from build123d import *

# Parameters (mm, degrees)
SKETCH1_W       = 34.29
SKETCH1_H       = 34.29
EXTRUDE1_DEPTH  = 1.27
SKETCH2_R       = 1.27
EXTRUDE2_DEPTH  = 2.27
SKETCH3_R       = 0.9525
EXTRUDE3_DEPTH  = 2.27
SKETCH4_R       = 0.5715
EXTRUDE4_DEPTH  = 2.27
LPATTERN1_COUNT = 3
LPATTERN1_PITCH = 2.54
SKETCH5_R       = 0.508
EXTRUDE5_DEPTH  = 2.27
LPATTERN2_COUNT = 8
LPATTERN2_PITCH = 2.54
SKETCH7_W       = 7.030885781
SKETCH7_H       = 5.062237762
SKETCH7_W_2     = 7.874
SKETCH7_H_2     = 7.62
SKETCH7_W_3     = 3.281080031
SKETCH7_H_3     = 6.374669774
SKETCH7_W_4     = 3.421697746
SKETCH7_H_4     = 4.921620047
SKETCH7_W_5     = 2.577991453
SKETCH7_H_5     = 1.453049728
SKETCH7_W_6     = 3.140462315
SKETCH7_H_6     = 1.406177157
SKETCH7_W_7     = 3.327952603
SKETCH7_H_7     = 1.078069153
EXTRUDE7_DEPTH  = 1.27
SKETCH8_R       = 3.175
EXTRUDE8_DEPTH  = 5.08
SKETCH9_W       = 7.112
SKETCH9_H       = 8.89
EXTRUDE9_DEPTH  = 2.54


with BuildPart() as part:
    # Sketch1 → Extrude1 (new body)
    with BuildSketch(Plane.XY):
        Rectangle(SKETCH1_W, SKETCH1_H)
    extrude(amount=EXTRUDE1_DEPTH)

    # Sketch2 → Extrude2 (cut, through all)
    with BuildSketch(Plane.XY.offset(1.27)):
        with Locations((-14.605, 14.605)):
            Circle(SKETCH2_R)
        with Locations((-14.605, -14.605)):
            Circle(SKETCH2_R)
        with Locations((14.605, -14.605)):
            Circle(SKETCH2_R)
    extrude(amount=-EXTRUDE2_DEPTH, mode=Mode.SUBTRACT)

    # Sketch3 → Extrude3 (cut, through all)
    with BuildSketch(Plane.XY.offset(1.27)):
        with Locations((-13.589, 0.762)):
            Circle(SKETCH3_R)
        with Locations((-13.589, -2.794)):
            Circle(SKETCH3_R)
        with Locations((-13.589, -6.35)):
            Circle(SKETCH3_R)
        with Locations((-13.589, -9.906)):
            Circle(SKETCH3_R)
    extrude(amount=-EXTRUDE3_DEPTH, mode=Mode.SUBTRACT)

    # Sketch4 → Extrude4 (cut, through all)
    with BuildSketch(Plane.XY.offset(1.27)):
        with Locations((6.35, -15.748)):
            Circle(SKETCH4_R)
        with Locations((8.89, -15.748)):
            Circle(SKETCH4_R)
    extrude4 = extrude(amount=-EXTRUDE4_DEPTH, mode=Mode.SUBTRACT)

    # LPattern1: Extrude4 ×3
    with Locations(*[(0, i * LPATTERN1_PITCH, 0) for i in range(1, LPATTERN1_COUNT)]):
        add(extrude4, mode=Mode.SUBTRACT)

    # Sketch5 → Extrude5 (cut, through all)
    with BuildSketch(Plane.XY.offset(1.27)):
        with Locations((15.367, -11.049)):
            Circle(SKETCH5_R)
    extrude5 = extrude(amount=-EXTRUDE5_DEPTH, mode=Mode.SUBTRACT)

    # LPattern2: Extrude5 ×8
    with Locations(*[(0, i * LPATTERN2_PITCH, 0) for i in range(1, LPATTERN2_COUNT)]):
        add(extrude5, mode=Mode.SUBTRACT)

    # Sketch7 → Extrude7 (add)
    with BuildSketch(Plane(origin=(0, 0, 0), x_dir=(-1, 0, 0), z_dir=(0, 0, -1))):
        with Locations((-8.390190366, 1.781157731)):
            Rectangle(SKETCH7_W, SKETCH7_H)
        with Locations((5.334, -9.525)):
            Rectangle(SKETCH7_W_2, SKETCH7_H_2)
        with Locations((1.640540016, 6.655905206)):
            Rectangle(SKETCH7_W_3, SKETCH7_H_3)
        with Locations((6.585596348, -0.210926574)):
            Rectangle(SKETCH7_W_4, SKETCH7_H_4)
        with Locations((-3.585751749, 11.64783411)):
            Rectangle(SKETCH7_W_5, SKETCH7_H_5)
        with Locations((1.992084305, 11.24941725)):
            Rectangle(SKETCH7_W_6, SKETCH7_H_6)
        with Locations((-10.241656955, -5.36690948)):
            Rectangle(SKETCH7_W_7, SKETCH7_H_7)
    extrude(amount=EXTRUDE7_DEPTH)

    # Sketch8 → Extrude8 (add)
    with BuildSketch(Plane(origin=(0, 0, 0), x_dir=(-1, 0, 0), z_dir=(0, 0, -1))):
        with Locations((8.509, 13.733663559)):
            Circle(SKETCH8_R)
        with Locations((12.827, 6.731)):
            Circle(SKETCH8_R)
    extrude(amount=EXTRUDE8_DEPTH)

    # Sketch9 → Extrude9 (add)
    with BuildSketch(Plane(origin=(0, 0, 0), x_dir=(-1, 0, 0), z_dir=(0, 0, -1))):
        with Locations((-10.795, 13.97)):
            Rectangle(SKETCH9_W, SKETCH9_H)
    extrude(amount=EXTRUDE9_DEPTH)


solid = part.part
Model file for the job. Use its own axes, mm. A direction names the side the tool comes from. Give positions to 0.01 mm unless a question says otherwise; leave off trailing zeros. Loops run counter-clockwise (first coordinate to the right, second up) from the corner with the lowest first, then second, coordinate; pieces in that order, holes last. Notation, with made-up numbers: (56.25, 89) -> (95.25, 89) arc R22 cw to (95.25, 128) -> close; hole circle Ø1 at (52, 15). An arc over 180 degrees is marked (long way). Use a Markdown table: item, result. Add a question column.
(1) Mould opens along X. For faces 6 (the cylindrical face through (14.964, 3.882, 0.644)), 7 (the flat face through (8, -0.75, -1)), 8 (the flat face through (11.906, 2, -1)) say: +X half, -X half, draft (parallel to the pull), parting line (faces both ways), or undercut.
(2) Wall check: line 1 along Y through (x, z) = (6.35, 0.75) (1 decimal); line 2 along X through (y, z) = (14.5, 0.75) (3 decimals); line 3 along Y through (x, z) = (-15, 0.75) (3 decimals). Give the ranges that are in metal, low to high.
(3) Slice it at B-B on x = -4. List the corners of the cut face in (y, z) (3 decimals), and give its area (3 significant figures).
(4) Tool access for faces 1 (the flat face through (2.297, 12, -1)), 2 (the flat face through (-5, -9, -1.27)), 3 (the flat face through (7.239, 14, -1)), 4 (the flat face through (4, 10.921, -1)), 5 (the flat face through (10, -4.828, -1)): list every direction of +Z, -Z, +X, -X, +Y, -Y with a clear straight run to the whole face (end or side of a thin tool).
(5) Slice it at A-A on x = 6.35. List the corners of the cut face in (y, z) (1 decimal), and give its area (3 significant figures).
(6) Drop flat-ended pins along their axis: pin 1 Ø2 at (x, z) = (-7, -4) entering from +Y; pin 2 Ø0.8 at (y, z) = (14, -1) entering from -X; pin 3 Ø10 at (x, y) = (9.5, -5.5) entering from -Z. Give the stop position or say it passes through.
(7) Slice it at C-C on x = -14. Give the number of separate pieces and of enclosed holes in the cut face, and give its area (3 significant figures).
(8) Slice it at D-D on z = -3.75. List the corners of the cut face in (x, y) (3 decimals), and give its area (3 significant figures).
Filled sheet:
| question | item | result |
|---|---|---|
| 1 | face 6 | undercut |
| 1 | face 7 | draft |
| 1 | face 8 | +X half |
| 2 | line 1 | -17.1 to -16.3, -15.2 to -13.8, -12.6 to -11.2, -10.1 to 17.1 |
| 2 | line 2 | -17.145 to -15.871, -13.339 to 17.145 |
| 2 | line 3 | -17.145 to -15.812, -13.398 to 13.398, 15.812 to 17.145 |
| 3 | outline | (-17.145, 0) -> (-13.335, 0) -> (-13.335, -1.27) -> (-5.715, -1.27) -> (-5.715, 0) -> (17.145, 0) -> (17.145, 1.27) -> (-17.145, 1.27) -> close |
| 3 | area | 53.2 mm2 |
| 4 | face 1 | -Z, +Y, -Y |
| 4 | face 2 | -Z, +X, -X, -Y |
| 4 | face 3 | -Z, +Y |
| 4 | face 4 | -Z, -Y |
| 4 | face 5 | -Z, +X, -X |
| 5 | outline | (-17.1, 0) -> (-16.3, 0) -> (-16.3, 1.3) -> (-17.1, 1.3) -> close; (-15.2, 0) -> (-13.8, 0) -> (-13.8, 1.3) -> (-15.2, 1.3) -> close; (-12.6, 0) -> (-11.2, 0) -> (-11.2, 1.3) -> (-12.6, 1.3) -> close; (-10.1, 0) -> (-0.7, 0) -> (-0.7, -1.3) -> (4.3, -1.3) -> (4.3, 0) -> (17.1, 0) -> (17.1, 1.3) -> (-10.1, 1.3) -> close |
| 5 | area | 45.6 mm2 |
| 6 | pin 1 | y = 16.87 |
| 6 | pin 2 | x = -11.68 |
| 6 | pin 3 | z = -1.27 |
| 7 | separate pieces | 7 |
| 7 | enclosed holes | 0 |
| 7 | area | 59.1 mm2 |
| 8 | outline | circle Ø6.35 at (-12.827, 6.731); circle Ø6.35 at (-8.509, 13.734) |
| 8 | area | 63.3 mm2 |
